For this review, use the dimensioned drawing (mm, ordinates from the lowest corner) and the shaded views. A direction names the side the tool comes from. Give positions to 0.01 mm unless a question says otherwise; leave off trailing zeros. Write each loop counter-clockwise with the first axis right and the second up, starting at its lowest first coordinate (ties: lowest second). Pieces come first, ordered by that corner, then holes.
1) We need section A-A on z = 10. Give the boundary of the cut face in (x, y), and give its area (3 significant figures).
2) We need section B-B on x = 10. Give the boundary of the cut face in (y, z).
3) We need section C-C on y = 65.5. Give the boundary of the cut face in (x, z).
4) We need section D-D on x = 18.25. Give the boundary of the cut face in (y, z).
5) Machinability: for the marked faces 1 and 2, which of the approach directions +Z, -Z, +X, -X, +Y, -Y give a long, thin tool a straight path to every point of the face, cutting with its end or side? Answer none if there is none.
6) For P1, Ø1, axis at x = 4, y = 62, coming from the -Z side; P2, Ø3, axis at y = 63.5, z = 14.5, coming from the -X side; P3, Ø12, axis at y = 18, z = 9, coming from the -X side, all flat-tipped, find the tip position at first contact; note any pin that passes through.
7) Wall thickness on line 1 along Y through (x, z) = (1.5, 18.25); line 2 along X through (y, z) = (55, 4); line 3 along Z through (x, y) = (5.75, 48.5): over which ranges is each line inside the solid? List them lowest first.
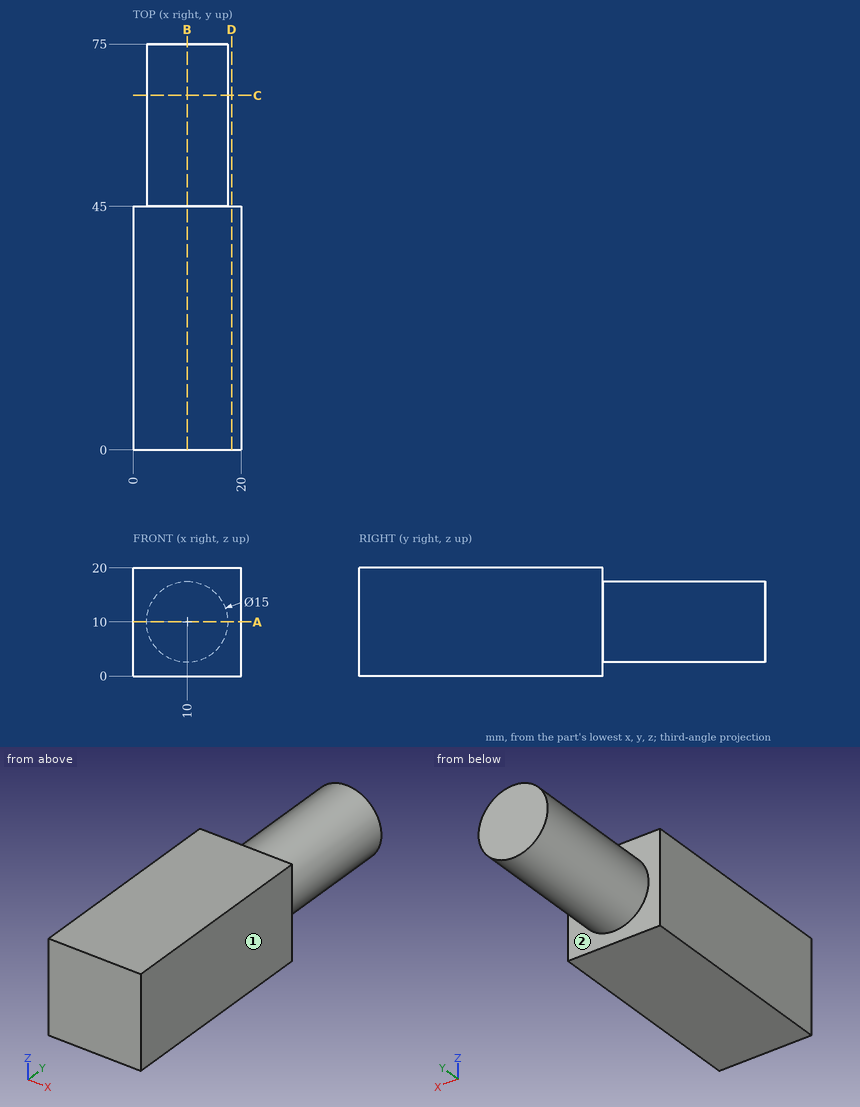
Results list:
1. outline: (0, 0) - (20, 0) - (20, 45) - (17.5, 45) - (17.5, 75) - (2.5, 75) - (2.5, 45) - (0, 45) - close
1. area: 1,350 mm2
2. outline: (0, 0) - (45, 0) - (45, 2.5) - (75, 2.5) - (75, 17.5) - (45, 17.5) - (45, 20) - (0, 20) - close
3. outline: circle Ø15 at (10, 10)
4. outline: (0, 0) - (45, 0) - (45, 20) - (0, 20) - close
5. face 1: +Z, -Z, +X, +Y, -Y
5. face 2: +Y
6. P1: stops at z = 4.9
6. P2: stops at x = 3.13
6. P3: stops at x = 0
7. line 1: y = 0 to 45
7. line 2: x = 5.5 to 14.5
7. line 3: z = 3.82 to 16.18
